Here's how the part is built. I have some questions about the finished solid (model axes, mm). Give positions to 0.01 mm unless a question says otherwise; leave off trailing zeros. Loops run counter-clockwise (first coordinate to the right, second up) from the corner with the lowest first, then second, coordinate; pieces in that order, holes last. Notation, with made-up numbers: (24, -20) -> (76, -20) arc R13 cw to (76, -4) -> close; hole circle Ø5 at (76.5, -34.5). An arc over 180 degrees is marked (long way). Answer in a Markdown table with one row per item. Add a question column.
Item 1: If we section it at C-C (y = 1.25): Write out the boundary of the cut face in (x, z), then the cut area to 3 significant figures.
Item 2: We'd pull the mould along Z, two halves only. Please class faces 1 (the face through (0.57, 3.04, -0.6)), 2 (the face through (37.3, 3, -4)), 3 (the face through (36.13, 2.96, -34.84)), 4 (the face through (11, 6, -35)): released by +Z, released by -Z, zero draft, split by the parting line, or undercut.
Item 3: If I drill on line 1 (X direction, y = 3.85, z = -5.5); line 2 (Z direction, x = 36.5, y = 2.85); line 3 (X direction, y = 4.5, z = -21), over which ranges is the centre line in solid material (lowest first)?
Item 4: If we section it at B-B (z = -30): Write out the boundary of the cut face in (x, y), then the cut area to 3 significant figures.
Item 5: If we section it at D-D (x = 12): Write out the boundary of the cut face in (y, z).
Item 6: If we section it at A-A (x = 5.5): Write out the boundary of the cut face in (y, z), then the cut area to 3 significant figures.
Item 7: For P1, Ø2.5, axis at x = 5.5, z = -5.5, coming from the +Y side; P2, Ø4, axis at x = 5.5, z = -36.5, coming from the +Y side, each with a flat end and sliding along its axis, tell me the tip position at first contact or that it passes through.
```python
from build123d import *

# Parameters (mm, degrees)
SKETCH_1_W                 = 42
SKETCH_1_H                 = 42
SKETCH_1_R                 = 15
EXTRUDE_1_DEPTH            = 6
FILLET_1_R                 = 2
HOLE_WIZARD_M3_1_OUTLINE_R = 1.7
HOLE_WIZARD_M3_1_DEPTH     = 6


# Read off the part's stored shape, not the designer's step: M3 间隙孔1
with BuildPart() as part:
    # 草图1 → 凸台-拉伸1 (new body)
    with BuildSketch(Plane(origin=(0, 0, 0), x_dir=(1, 0, 0), z_dir=(0, 1, 0))):
        with Locations((21, 21)):
            Rectangle(SKETCH_1_W, SKETCH_1_H)
        with Locations(Location((21, 21, 0), (0, 0, 270))):
            Circle(SKETCH_1_R, mode=Mode.SUBTRACT)
    extrude(amount=EXTRUDE_1_DEPTH)

    # 圆角1
    fillet_1_edges = [part.edges().sort_by_distance(p)[0] for p in [
        (0, 3, -42),
        (42, 3, -42),
        (42, 3, 0),
        (0, 3, 0),
    ]]
    fillet(fillet_1_edges, radius=FILLET_1_R)

    # M3 间隙孔1 outline → M3 间隙孔1 (cut)
    with BuildSketch(Plane(origin=(0, 0, 0), x_dir=(1, 0, 0), z_dir=(0, 1, 0))):
        with Locations((36.5, 36.5)):
            Circle(HOLE_WIZARD_M3_1_OUTLINE_R)
        with Locations((5.5, 5.5)):
            Circle(HOLE_WIZARD_M3_1_OUTLINE_R)
        with Locations((36.5, 5.5)):
            Circle(HOLE_WIZARD_M3_1_OUTLINE_R)
        with Locations((5.5, 36.5)):
            Circle(HOLE_WIZARD_M3_1_OUTLINE_R)
    extrude(amount=HOLE_WIZARD_M3_1_DEPTH, mode=Mode.SUBTRACT)


solid = part.part
```
Recorded:
| question | item | result |
|---|---|---|
| 1 | outline | (0, -40) arc R2 ccw to (2, -42) -> (40, -42) arc R2 ccw to (42, -40) -> (42, -2) arc R2 ccw to (40, 0) -> (2, 0) arc R2 ccw to (0, -2) -> close; hole circle Ø3.4 at (5.5, -36.5); hole circle Ø3.4 at (5.5, -5.5); hole circle Ø30 at (21, -21); hole circle Ø3.4 at (36.5, -36.5); hole circle Ø3.4 at (36.5, -5.5) |
| 1 | area | 1,020 mm^2 |
| 2 | face 1 | released by +Z |
| 2 | face 2 | undercut |
| 2 | face 3 | undercut |
| 2 | face 4 | zero draft |
| 3 | line 1 | x = 0 to 3.8, 7.2 to 34.8, 38.2 to 42 |
| 3 | line 2 | z = -42 to -38.2, -34.8 to -7.2, -3.8 to 0 |
| 3 | line 3 | x = 0 to 6, 36 to 42 |
| 4 | outline | (0, 0) -> (9, 0) -> (9, 6) -> (0, 6) -> close; (33, 0) -> (42, 0) -> (42, 6) -> (33, 6) -> close |
| 4 | area | 108 mm^2 |
| 5 | outline | (0, -42) -> (6, -42) -> (6, -33) -> (0, -33) -> close; (0, -9) -> (6, -9) -> (6, 0) -> (0, 0) -> close |
| 6 | outline | (0, -42) -> (6, -42) -> (6, -38.2) -> (0, -38.2) -> close; (0, -34.8) -> (6, -34.8) -> (6, -7.2) -> (0, -7.2) -> close; (0, -3.8) -> (6, -3.8) -> (6, 0) -> (0, 0) -> close |
| 6 | area | 211 mm^2 |
| 7 | P1 | passes through |
| 7 | P2 | stops at y = 6 |
